Here's the drawing with two shaded views (mm, measured from the low corner). I have some questions. A direction names the side the tool comes from. Give positions to 0.01 mm unless a question says otherwise; leave off trailing zeros. Write each loop counter-clockwise with the first axis right and the second up, starting at its lowest first coordinate (ties: lowest second). Pieces come first, ordered by that corner, then holes.
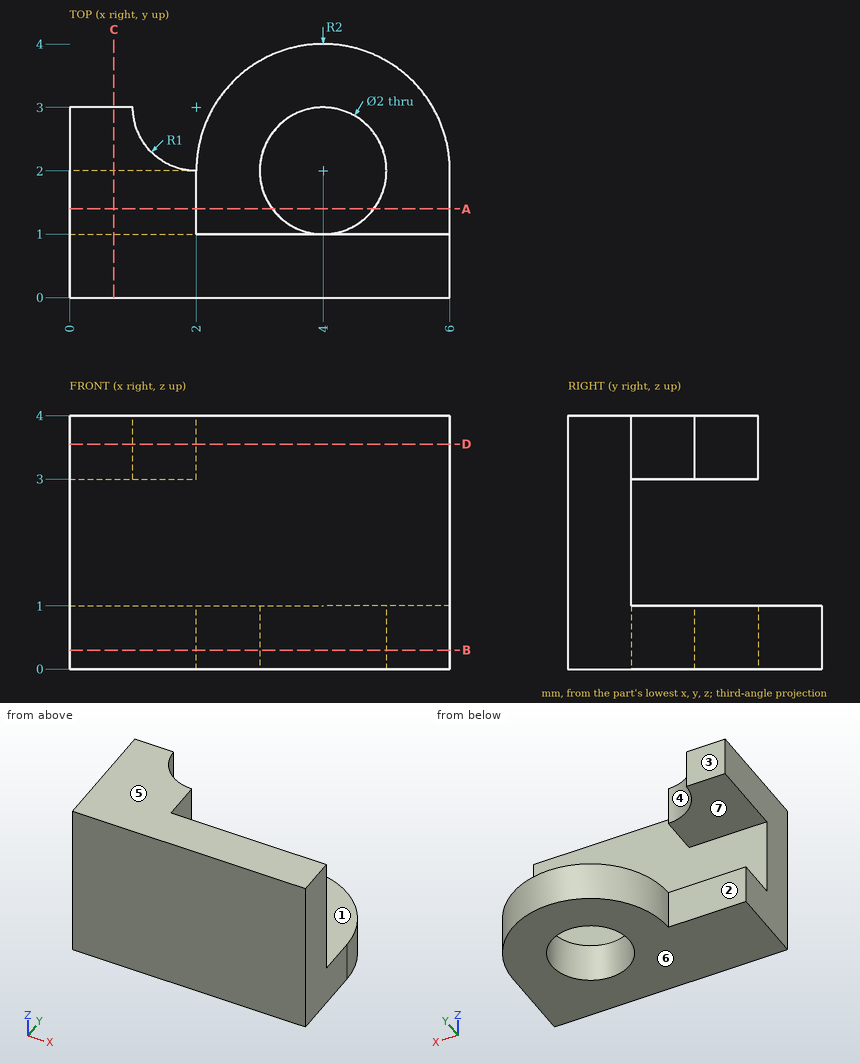
(1) Imagine slicing it at D-D, the plane z = 3.55. Write out the boundary of the cut face in (x, y), plus the area to 3 significant figures.
Returned:
outline: (0, 0) - (6, 0) - (6, 1) - (2, 1) - (2, 2) arc R1 cw to (1, 3) - (0, 3) - close
area: 9.21 mm2
(2) If we mould it in two halves opening along Z, with no side actions, what happens to the marked faces 4, 5, 6 and 7? For each: +Z half, -Z half, draft (parallel to the pull), parting line (faces both ways), or undercut.
Returned:
face 4: draft
face 5: +Z half
face 6: -Z half
face 7: undercut
(3) Imagine slicing it at B-B, the plane z = 0.3. Write out the boundary of the cut face in (x, y).
Returned:
outline: (0, 0) - (6, 0) - (6, 2) arc R2 ccw to (2, 2) - (0, 2) - close; hole circle Ø2 at (4, 2)
(4) For the marked faces 1, 2 and 3, which set-ups out of +Z, -Z, +X, -X, +Y, -Y let a thin tool reach every point of the face, with its end or its side?
Returned:
face 1: +X, -X, +Y
face 2: -Z, -X, +Y
face 3: +Z, -Z, +X, -X, +Y
(5) If I drill on L1, parallel to Y at x = 4, z = 0.6; L2, parallel to Z at x = 4.5, y = 3.7, over which ranges is the centre line in solid material (lowest first)?
Returned:
L1: y = 0 to 1, 3 to 4
L2: z = 0 to 1
(6) Will this pin go through, and if not, where does the flat tip stop? P1, Ø1.5, axis at x = 1.5, y = 3.5, coming from the -Z side.
Returned:
P1: stops at z = 3
(7) Imagine slicing it at A-A, the plane y = 1.4. Write out the boundary of the cut face in (x, z), plus the area to 3 significant figures.
Returned:
outline: (0, 0) - (3.2, 0) - (3.2, 1) - (0, 1) - close; (0, 3) - (2, 3) - (2, 4) - (0, 4) - close; (4.8, 0) - (6, 0) - (6, 1) - (4.8, 1) - close
area: 6.40 mm2
(8) Imagine slicing it at C-C, the plane x = 0.7. Write out the boundary of the cut face in (y, z), plus the area to 3 significant figures.
Returned:
outline: (0, 0) - (2, 0) - (2, 1) - (1, 1) - (1, 3) - (3, 3) - (3, 4) - (0, 4) - close
area: 7.00 mm2
